Geometry: final body of the model. Coordinates: model frame, mm. Give positions to 0.01 mm unless a question says otherwise; leave off trailing zeros. Write each loop counter-clockwise with the first axis right and the second up, starting at its lowest first coordinate (ties: lowest second). Pieces come first, ordered by that corner, then holes. Notation, with made-up numbers: (1, 87.25) - (30, 87.25) arc R14 cw to (30, 101.25) - close; hole circle Ø6 at (65.5, -16). An arc over 180 degrees is marked (long way). Return JSON: item names as keys, results as strings.
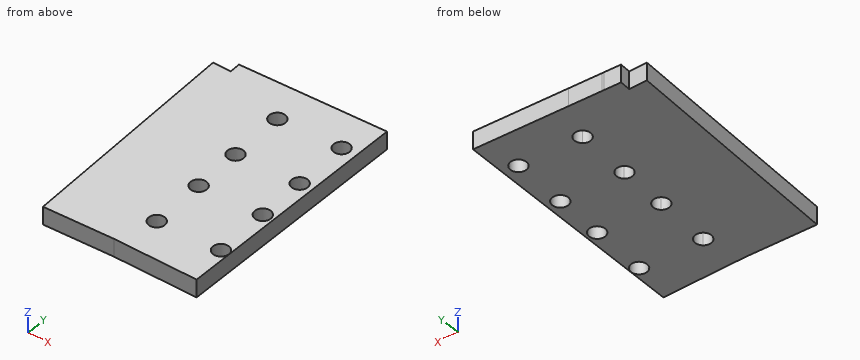
Autodesk Inventor part; units mm, degrees
ref_plane "YZ Plane" through (0, 0, 0) normal (1, 0, 0) x (0, 1, 0)
ref_plane "XZ Plane" through (0, 0, 0) normal (0, 1, 0) x (-1, 0, 0)
ref_plane "XY Plane" through (0, 0, 0) normal (0, 0, 1) x (1, 0, 0)
sketch "Skizze1" plane through (0, 0, 0) normal (0, 0, 1) x (1, 0, 0)
  ellipse E0 centre (-12.1961, -42.2319) end of major axis (-9.6527, -42.1265) minor radius 1.8 (-13.7003, -43.7155) -> (-13.818, -40.878) ccw
  arc A0 (-13.818, -40.878) -> (-13.7003, -43.7155) centre (-14.8644, -42.3426) ccw
  ellipse E1 centre (-12.6519, -31.2414) end of major axis (-10.1085, -31.1359) minor radius 1.8 (-14.1561, -32.725) -> (-14.2737, -29.8874) ccw
  arc A1 (-14.2737, -29.8874) -> (-14.1561, -32.725) centre (-15.3201, -31.352) ccw
  ellipse E2 centre (-13.1697, -18.7521) end of major axis (-10.6263, -18.6467) minor radius 1.8 (-14.6739, -20.2357) -> (-14.7916, -17.3982) ccw
  arc A2 (-14.7916, -17.3982) -> (-14.6739, -20.2357) centre (-15.838, -18.8628) ccw
  ellipse E3 centre (-11.6782, -54.7212) end of major axis (-9.1348, -54.6157) minor radius 1.8 (-13.1824, -56.2048) -> (-13.3001, -53.3673) ccw
  arc A3 (-13.3001, -53.3673) -> (-13.1824, -56.2048) centre (-14.3465, -54.8319) ccw
  line L0 (1.4946, -9.6367) -> (3.6905, -62.5912)
  line L1 (1.4946, -9.6367) -> (-19.2875, -10.4985)
  line L2 (-19.2875, -10.4985) -> (-17.0916, -63.453)
  line L3 (-17.0916, -63.453) -> (3.6905, -62.5912)
  circle A4 centre (-0.8764, -41.7626) radius 1.8
  circle A5 centre (-1.3321, -30.772) radius 1.8
  circle A6 centre (-1.85, -18.2827) radius 1.8
  circle A7 centre (-0.3585, -54.2518) radius 1.8
  line L4 (1.4946, -9.6367) -> (-17.0916, -9.6367)
  line L5 (-17.0916, -9.6367) -> (-17.0916, -63.453)
  line L6 (-17.0916, -63.453) -> (1.4946, -63.453)
  line L7 (1.4946, -63.453) -> (1.4946, -9.6367)
  circle A8 centre (-0.3585, -54.2518) radius 1.8
  circle A9 centre (-0.8764, -41.7626) radius 1.8
  circle A10 centre (-1.3321, -30.772) radius 1.8
  circle A11 centre (-1.85, -18.2827) radius 1.8
  circle A12 centre (-15.838, -18.8628) radius 1.8
  circle A13 centre (-15.3201, -31.352) radius 1.8
  circle A14 centre (-14.8644, -42.3426) radius 1.8
  circle A15 centre (-14.3465, -54.8319) radius 1.8
  point P0 (0, 0)
extrude "Extrusion1" add sketch "Skizze1" along normal blind 4 contours A14 E0 | A13 E1 | E1 A1 L5 A2 E2 L1 L7 L3 | L5 L2 L1 A2 A1 | L3 L7 L6 | A12 E2 | A15 E3
sketch "Skizze2" plane through (1.4946, -9.6367, 0) normal (1, 0, 0) x (0, 0, 1)
  line L0 (0, 0.8618) -> (0, 53.8163)
  line L1 (0, 0.8618) -> (19, 0.8618)
  line L2 (19, 0.8618) -> (19, 53.8163)
  line L3 (19, 53.8163) -> (0, 53.8163)
  line L4 (0, 53.8163) -> (0, 0.8618)
  line L5 (4, 53.8163) -> (4, 0)
  point P0 (0, -9.6367)
  dimension "d3" = 15
extrude "Extrusion2" [suppressed]
sketch "Skizze3" plane through (-6.3, -26.5, 0) normal (1, 0, 0) x (0, 0, -1)
  line L0 (-7, 52) -> (-15, 52)
  line L1 (-15, 52) -> (-15, 35)
  line L2 (-15, 35) -> (-7, 35)
  line L3 (-7, 35) -> (-7, 52)
  line L4 (-4, 53) -> (-4, 0)
  line L5 (-19, 53) -> (-4, 53)
  circle A0 centre (-11, 31) radius 1.5
  point P0 (0, 26.5)
  dimension "d6" = 8
  dimension "d7" = 17
  dimension "d8" = 3
  dimension "d9" = 1
  dimension "d10" = 4
  dimension "d11" = 3
  dimension "d12" = 4
extrude "Extrusion3" [suppressed]
ref_plane "Arbeitsebene1" through (-1296.3098, -63.453, 4) normal (0.0207202, -0.9997853, 0) x (0, 0, 1)
mirror "Spiegeln1" [suppressed]
sketch "Skizze4" plane through (-19.2875, -10.4985, 0) normal (-0.9991413, -0.0414316, 0) x (0, 0, -1)
  line L0 (0, 0) -> (0, 53)
  line L1 (0, 53) -> (-4, 53)
  line L2 (-4, 0) -> (-4, 53)
  line L3 (0, 0) -> (-4, 0)
  point P0 (0, -9.6904)
extrude "Extrusion4" add sketch "Skizze4" along normal blind 15.5
sketch "Skizze5" plane through (0, 0, 4) normal (0, 0, 1) x (1, 0, 0)
  line L0 (-30.6781, -13.3745) -> (-38.5781, -13.3745)
  line L1 (-38.5781, -13.3745) -> (-39.6071, 11.4403)
  line L2 (-39.6071, 11.4403) -> (-31.7139, 11.6041)
  line L3 (-31.7139, 11.6041) -> (-30.6781, -13.3745)
  line L4 (-32.5783, -64.0952) -> (-34.7742, -11.1407)
  line L5 (-17.0916, -63.453) -> (-32.5783, -63.453)
  line L6 (1.4946, -9.6367) -> (-34.7742, -11.1407)
  circle A0 centre (-26.901, -9.1245) radius 1.7
  circle A1 centre (-28.2889, 24.3468) radius 1.7
  point P0 (0, 0)
  point P1 (-6.3, 26.5)
  point P2 (-6.3, -26.5)
  point P3 (1.4946, -9.6367)
  dimension "d26" = 7.9
  dimension "d27" = 25
  dimension "d28" = 14
  dimension "d29" = 53
  dimension "d30" = 3.95
  dimension "d31" = 3.95
  dimension "d32" = 33.5
  dimension "d33" = 3.4
  dimension "d34" = 3.4
  dimension "d35" = 4.25
  dimension "d41" = 4
extrude "Extrusion5" cut sketch "Skizze5" against normal blind 4
equation "\"d12\" = 0.5 * d6"
equation "\"d28\" = -0.5 * d27 + 0.5 * d29"
equation "\"d30\" = 0.5 * d26"
equation "\"d31\" = d30"
equation "\"d34\" = d33"
equation "\"d35\" = 0.5 * d32 - 0.5 * d27"
properties part number "cable_mount"
Q1. Pin query (flat end, axial travel): P1, Ø4.5, axis at x = -14.35, y = -54.83, coming from the -Z side; P2, Ø2, axis at x = -15.84, y = -18.86, coming from the +Z side; P3, Ø2, axis at x = -32.5, z = 3, coming from the +Y side. Return the tip coordinate at first contact, or that it passes through.
Answer key:
{"P1": "stops at z = 0", "P2": "passes through", "P3": "stops at y = -13.37"}
Q2. Section query C-C, the plane x = -24.5. Return the cut outline in (y, z).
Answer key:
{"outline": "(-63.76, 0) - (-10.71, 0) - (-10.71, 4) - (-63.76, 4) - close"}
Q3. Section query A-A, the plane y = -19. Return the cut outline in (x, z).
Answer key:
{"outline": "(-34.45, 0) - (-17.63, 0) - (-17.63, 4) - (-34.45, 4) - close; (-14.04, 0) - (-3.5, 0) - (-3.5, 4) - (-14.04, 4) - close; (-0.2, 0) - (1.49, 0) - (1.49, 4) - (-0.2, 4) - close"}
Q4. Section query D-D, the plane y = -47. Return the cut outline in (x, z).
Answer key:
{"outline": "(-33.29, 0) - (1.49, 0) - (1.49, 4) - (-33.29, 4) - close"}
Q5. Material intervals for probe 1 along X at (y, z) = (-30, 0.2); probe 2 along Y at (x, z) = (-1.5, 3.1); probe 3 along X at (y, z) = (-30.5, 2.3), sorted ascending. Write a range as [from, to].
Answer key:
{"probe 1": "x = [-33.99, -16.51], [-14.13, -2.96], [0.29, 1.49]", "probe 2": "y = [-63.45, -55.64], [-52.86, -43.45], [-40.07, -32.56], [-28.98, -20.05], [-16.52, -9.76]", "probe 3": "x = [-33.97, -16.91], [-13.73, -3.11], [0.45, 1.49]"}
Q6. Section query B-B, the plane z = 3.4. Count the separate pieces of the cut face and the enclosed holes in it, plus the area to 3 significant figures.
Answer key:
{"separate pieces": "1", "enclosed holes": "8", "area": "1,780 mm^2"}
